from build123d import *

# Parameters (mm, degrees)
SKETCH_1_R      = 4
SKETCH_1_R_2    = 10
SKETCH_1_R_3    = 5
SKETCH_1_R_4    = 9
EXTRUDE_1_DEPTH = 10
SKETCH_1_3_R    = 33
SKETCH_1_3_R_2  = 10
SKETCH_1_3_R_3  = 3
EXTRUDE_2_DEPTH = 20


with BuildPart() as part:
    # Sketch 1 → Extrude 1 (new body)
    with BuildSketch(Plane.XY):
        with BuildLine():
            Line((-134, 75), (-188, 75))
            Line((-188, 75), (-188, 56.479823981))
            ThreePointArc((-188, 56.479823981), (-186.980113599, 52.571113945), (-184.180496463, 49.659013961))
            Line((-184.180496463, 49.659013961), (-126, 14))
            Line((-126, 14), (-90, 14))
            ThreePointArc((-90, 14), (-76, 0), (-90, -14))
            Line((-90, -14), (-126, -14))
            Line((-126, -14), (-184.180496463, -49.659013961))
            ThreePointArc((-184.180496463, -49.659013961), (-186.980113599, -52.571113945), (-188, -56.479823981))
            Line((-188, -56.479823981), (-188, -75))
            Line((-188, -75), (-134, -75))
            ThreePointArc((-134, -75), (-128.343145751, -72.656854249), (-126, -67))
            Line((-126, -67), (-126, -60))
            ThreePointArc((-126, -60), (-123.656854249, -54.343145751), (-118, -52))
            Line((-118, -52), (-90, -52))
            ThreePointArc((-90, -52), (-68.657428628, -47.418294436), (-51.075833333, -34.480563355))
            ThreePointArc((-51.075833333, -34.480563355), (-34.708861379, -25.426163433), (-16.292622951, -28.697568493))
            ThreePointArc((-16.292622951, -28.697568493), (-33, 0), (-16.292622951, 28.697568493))
            ThreePointArc((-16.292622951, 28.697568493), (-34.708861379, 25.426163433), (-51.075833333, 34.480563355))
            ThreePointArc((-51.075833333, 34.480563355), (-68.657428628, 47.418294436), (-90, 52))
            Line((-90, 52), (-118, 52))
            ThreePointArc((-118, 52), (-123.656854249, 54.343145751), (-126, 60))
            Line((-126, 60), (-126, 67))
            ThreePointArc((-126, 67), (-128.343145751, 72.656854249), (-134, 75))
        make_face()
        with Locations((-173, -59)):
            Circle(SKETCH_1_R, mode=Mode.SUBTRACT)
        with Locations((-148, -59)):
            Circle(SKETCH_1_R_2, mode=Mode.SUBTRACT)
        with Locations((-69, -15.588457268)):
            Circle(SKETCH_1_R_3, mode=Mode.SUBTRACT)
        with Locations((-173, 59)):
            Circle(SKETCH_1_R, mode=Mode.SUBTRACT)
        with Locations((-148, 59)):
            Circle(SKETCH_1_R_2, mode=Mode.SUBTRACT)
        with Locations((-60, 0)):
            Circle(SKETCH_1_R_4, mode=Mode.SUBTRACT)
        with Locations((-69, 15.588457268)):
            Circle(SKETCH_1_R_3, mode=Mode.SUBTRACT)
        with Locations((-42, 0)):
            Circle(SKETCH_1_R_3, mode=Mode.SUBTRACT)
    extrude(amount=EXTRUDE_1_DEPTH)

    # Sketch 1_3 → Extrude 2 (add)
    with BuildSketch(Plane.XY):
        with Locations(Location((0, 0, 0), (0, 0, 240.414892568))):
            Circle(SKETCH_1_3_R)
        Circle(SKETCH_1_3_R_2, mode=Mode.SUBTRACT)
        with Locations((-16.180339887, 11.755705046)):
            Circle(SKETCH_1_3_R_3, mode=Mode.SUBTRACT)
        with Locations((-16.180339887, -11.755705046)):
            Circle(SKETCH_1_3_R_3, mode=Mode.SUBTRACT)
        with Locations((6.180339887, -19.021130326)):
            Circle(SKETCH_1_3_R_3, mode=Mode.SUBTRACT)
        with Locations((20, 0)):
            Circle(SKETCH_1_3_R_3, mode=Mode.SUBTRACT)
        with Locations((6.180339887, 19.021130326)):
            Circle(SKETCH_1_3_R_3, mode=Mode.SUBTRACT)
    extrude(amount=EXTRUDE_2_DEPTH)


solid = part.part
The listing builds one solid part. Answer for the finished solid, in the listing's coordinates (mm). A direction names the side the tool comes from. Coordinates: 2 decimals unless noted, no trailing zeros. Loops run counter-clockwise (first coordinate to the right, second up) from the corner with the lowest first, then second, coordinate; pieces in that order, holes last.
1) Find section C-C on z = 16. Write down the section's boundary in (x, y), then the cut area to 3 significant figures.
2) Find section A-A on x = 0. Write down the section's boundary in (y, z).
3) Find section D-D on x = -97.5. Write down the section's boundary in (y, z).
4) A tool of negligible diameter and unlimited length cuts with its end or side. For faces 4 (the face through (-104, -52, 5)), 5 (the face through (-171.154, -62.549, 4.93)), 6 (the face through (-155.5, 32.08, 4.93)), from which of +Z, -Z, +X, -X, +Y, -Y can it reach the whole face along a straight path? Write none if from no direction.
5) Find section B-B on x = -173. Write down the section's boundary in (y, z), then the cut area to 3 significant figures.
6) Determine the mould class of faces 1 (the face through (-47, 0, 5)), 2 (the face through (-71, 9, 0)), 3 (the face through (-123.594, 54.281, 4.93)) for opening direction Y: pulls with the +Y half, pulls with the -Y half, needs draft (parallel to the pull), parting line crosses it, or undercut.
7) Find the intervals of material crossed by L1, parallel to Y at x = 0, z = 13.5; L2, parallel to Y at x = -70.5, z = 1.25; L3, parallel to Y at x = -173, z = 3.25, in increasing order.
8) Flat-ended cylindrical pins translate along their axes: pin 1 Ø5.5 at (x, y) = (-16.18, 11.76) entering from +Z (1 decimal); pin 2 Ø8 at (x, z) = (-64, 6) entering from -Y; pin 3 Ø6 at (y, z) = (-33.5, 3) entering from +X; pin 4 Ø8 at (x, z) = (-99, 6.5) entering from -Y. Find the tip coordinate at first contact, or state that the pin passes through.
Values:
1. outline: circle Ø66 at (0, 0); hole circle Ø6 at (-16.18, -11.76); hole circle Ø6 at (-16.18, 11.76); hole circle Ø20 at (0, 0); hole circle Ø6 at (6.18, -19.02); hole circle Ø6 at (6.18, 19.02); hole circle Ø6 at (20, 0)
1. area: 2,970 mm2
2. outline: (-33, 0) - (-10, 0) - (-10, 20) - (-33, 20) - close; (10, 0) - (33, 0) - (33, 20) - (10, 20) - close
3. outline: (-52, 0) - (-14, 0) - (-14, 10) - (-52, 10) - close; (14, 0) - (52, 0) - (52, 10) - (14, 10) - close
4. face 4: +Z, -Z, +X, -Y
4. face 5: +Z, -Z
4. face 6: +Z, -Z, -X
5. outline: (-75, 0) - (-63, 0) - (-63, 10) - (-75, 10) - close; (-55, 0) - (-42.81, 0) - (-42.81, 10) - (-55, 10) - close; (42.81, 0) - (55, 0) - (55, 10) - (42.81, 10) - close; (63, 0) - (75, 0) - (75, 10) - (63, 10) - close
5. area: 484 mm2
6. face 1: undercut
6. face 2: needs draft
6. face 3: pulls with the +Y half
7. L1: y = -33 to -10, 10 to 33
7. L2: y = -48.21 to -20.36, -10.82 to 10.82, 20.36 to 48.21
7. L3: y = -75 to -63, -55 to -42.81, 42.81 to 55, 63 to 75
8. pin 1: passes through
8. pin 2: stops at y = -47.12
8. pin 3: stops at x = 12.6
8. pin 4: stops at y = -52
